Work out the finished part from the listing and answer in its coordinate system (mm). A direction names the side the tool comes from. Coordinates: 2 decimals unless noted, no trailing zeros. Order: outer loops, then holes, each group sorted by start corner. A loop starts at its lowest first (then second) coordinate and runs counter-clockwise, first axis right, second up. Notation, with made-up numbers: M 57.25,59 L 71.25,59 A21 cw 71.25,72 Z; hole C 35,56 d5. An arc over 180 degrees is marked long. Use a Markdown table: item, result.
from build123d import *

# Parameters (mm, degrees)
SKETCH2_R               = 2.000000064
BOSS_EXTRUDE2_DEPTH     = 3.175
SKETCH1_R               = 2.000000064
BOSS_EXTRUDE3_DEPTH     = 3.175
SKETCH3_R               = 2.000000064
CUT_EXTRUDE1_DEPTH      = 1
CUT_EXTRUDE1_DEPTH_BACK = 4.175


with BuildPart() as part:
    # Sketch2 → Boss-Extrude2 (new body)
    with BuildSketch(Plane(origin=(0, 0, 0), x_dir=(1, 0, 0), z_dir=(0, 1, 0))):
        with BuildLine():
            Line((-36.96683296, -6.1921984), (-96.411937598, 7.313398015))
            ThreePointArc((-96.411937598, 7.313398015), (-101.197303038, 14.912429375), (-93.598271679, 19.697794815))
            Line((-93.598271679, 19.697794815), (-34.15316704, 6.1921984))
            ThreePointArc((-34.15316704, 6.1921984), (-29.3678016, -1.40683296), (-36.96683296, -6.1921984))
        make_face()
        with Locations((-95.005104638, 13.505596415)):
            Circle(SKETCH2_R, mode=Mode.SUBTRACT)
    extrude(amount=BOSS_EXTRUDE2_DEPTH)

    # Sketch1 → Boss-Extrude3 (add)
    with BuildSketch(Plane(origin=(0, 0, 0), x_dir=(1, 0, 0), z_dir=(0, 1, 0))):
        with BuildLine():
            Line((-35.56, 6.35), (35.56, 6.35))
            ThreePointArc((35.56, 6.35), (41.91, 0), (35.56, -6.35))
            Line((35.56, -6.35), (-35.56, -6.35))
            ThreePointArc((-35.56, -6.35), (-41.91, 0), (-35.56, 6.35))
        make_face()
        with Locations((35.56, 0)):
            Circle(SKETCH1_R, mode=Mode.SUBTRACT)
    extrude(amount=BOSS_EXTRUDE3_DEPTH)

    # Sketch3 → Cut-Extrude1 (cut, two sides)
    with BuildSketch(Plane(origin=(0, 3.175, 0), x_dir=(1, 0, 0), z_dir=(0, 1, 0))) as cut_extrude1_sk:
        with Locations((-35.56, 0)):
            Circle(SKETCH3_R)
    extrude(amount=CUT_EXTRUDE1_DEPTH, mode=Mode.SUBTRACT)
    extrude(cut_extrude1_sk.sketch, amount=-CUT_EXTRUDE1_DEPTH_BACK, mode=Mode.SUBTRACT)


solid = part.part
(1) A cutting plane is placed at A-A (z = 0). Determine the outline of the cut face in (x, y) (3 decimals), then the cut area to 3 significant figures.
Conclusion:
| item | result |
|---|---|
| outline | M -64.222,0 L -37.56,0 L -37.56,3.175 L -64.222,3.175 Z; M -33.56,0 L 33.56,0 L 33.56,3.175 L -33.56,3.175 Z; M 37.56,0 L 41.91,0 L 41.91,3.175 L 37.56,3.175 Z |
| area | 312 mm2 |
(2) A cutting plane is placed at B-B (y = 2.2). Determine the outline of the cut face in (x, z).
Conclusion:
| item | result |
|---|---|
| outline | M -96.41,-7.31 A6.35 ccw -93.6,-19.7 L -34.85,-6.35 L 35.56,-6.35 A6.35 ccw 35.56,6.35 L -35.56,6.35 A6.35 ccw -36.97,6.19 Z; hole C -95.01,-13.51 d4; hole C -35.56,0 d4; hole C 35.56,0 d4 |
(3) A cutting plane is placed at D-D (z = -16.75). Determine the outline of the cut face in (x, y) (1 decimal).
Conclusion:
| item | result |
|---|---|
| outline | M -100.5,0 L -80.6,0 L -80.6,3.2 L -100.5,3.2 Z |
(4) Given P1, Ø3.5, axis at x = -95.01, z = -13.51, coming from the +Y side; P2, Ø4.5, axis at x = 35.56, z = 0, coming from the +Y side (3 decimals); P3, Ø1.5, axis at x = -38.5, y = 2.5, coming from the +Z side, each flat-ended and moving along its own axis, determine where each tip first touches the part or whether it passes through.
Conclusion:
| item | result |
|---|---|
| P1 | through |
| P2 | y = 3.175 |
| P3 | z = 6.01 |
(5) Which of the six approach directions +Z, -Z, +X, -X, +Y, -Y give full straight-line access (tool end or side, diameter ignored) to faces 1 (the flat face through (0, 2, -6.35)), 2 (the flat face through (-29, 0, -4))?
Conclusion:
| item | result |
|---|---|
| face 1 | -Z, +X, +Y, -Y |
| face 2 | +Z, -Z, +X, -X, -Y |
(6) A cutting plane is placed at C-C (x = -77.5). Determine the outline of the cut face in (y, z) (3 decimals), then the cut area to 4 significant figures.
Conclusion:
| item | result |
|---|---|
| outline | M 0,-16.04 L 3.175,-16.04 L 3.175,-3.017 L 0,-3.017 Z |
| area | 41.35 mm2 |
(7) Straight lines are drawn through the part: L1, parallel to Z at x = 35.56, y = 1.35; L2, parallel to Z at x = -35.56, y = 2.2; L3, parallel to Z at x = -16, y = 0.1. For each, find the intervals that lie inside material, in ascending order.
Conclusion:
| item | result |
|---|---|
| L1 | -6.35 to -2, 2 to 6.35 |
| L2 | -6.51 to -2, 2 to 6.35 |
| L3 | -6.35 to 6.35 |
(8) Determine the mould class of faces 3 (the cylindrical face through (33.562, 1.565, -0.088)), 4 (the flat face through (-64.634, 1.565, -13.117)), 5 (the cylindrical face through (-101.227, 1.565, -14.776)) for opening direction Z: pulls with the +Z half, pulls with the -Z half, needs draft (parallel to the pull), parting line crosses it, or undercut.
Conclusion:
| item | result |
|---|---|
| face 3 | undercut |
| face 4 | pulls with the -Z half |
| face 5 | parting line crosses it |
